Source: CAD feature listing. Evaluate the final solid. Frame: model axes, mm. A direction names the side the tool comes from. Round coordinates to 2 decimals unless told otherwise and drop trailing zeros. Loops run counter-clockwise (first coordinate to the right, second up) from the corner with the lowest first, then second, coordinate; pieces in that order, holes last. Notation, with made-up numbers: (55.5, -31) -> (90.5, -31) arc R38 cw to (90.5, 7) -> close; hole circle Ø6 at (38.25, 81). An arc over 180 degrees is marked (long way). Put each result on its own line as item: value. Start each with the question number.
1. Cut plane A-A (z = 0). Return the cut outline in (x, y), then the cut area to 3 significant figures.
2. Material intervals for L1, parallel to Y at x = 4, z = -4.5; L2, parallel to Z at x = 0, y = 53; L3, parallel to X at y = 32, z = 4.25, sorted ascending.
3. Draft query along Z for faces 1 (the flat face through (20.75, 2, 0)), 2 (the flat face through (10, 2, -10)), 3 (the flat face through (10, 4, 0)). Return one class per face: pulls with the +Z half, pulls with the -Z half, needs draft (parallel to the pull), parting line crosses it, or undercut.
4. Cut plane B-B (x = 0). Return the cut outline in (y, z).
5. Cut plane C-C (z = -7.75). Return the cut outline in (x, y), then the cut area to 3 significant figures.
6. Set-up query: faces 4 (the flat face through (27.25, 2, 0)), 5 (the cylindrical face through (-2.192, 31.608, 4.214)), 6 (the flat face through (16.75, 2, 0)). Return all of +Z, -Z, +X, -X, +Y, -Y with unobstructed straight access to the full face (end or side cutting, diameter ignored); none if empty.
7. Cut plane D-D (y = 8.5). Return the cut outline in (x, z).
8. Contact query for flat-ended pins moving along their axis: pin 1 (3 mm diameter, centred on y = 22, z = -1, fed in from +X); pin 2 (8 mm diameter, centred on x = 0.5, y = 9.5, fed in from -Z); pin 3 (2 mm diameter, centred on y = 47, z = -7.5, fed in from -X); pin 4 (6 mm diameter, centred on y = 43.5, z = -1.5, fed in from -X). Output: stop coordinate, or through.
Autodesk Inventor part; units mm, degrees
ref_plane "YZ Plane" through (0, 0, 0) normal (1, 0, 0) x (0, 1, 0)
ref_plane "XZ Plane" through (0, 0, 0) normal (0, 1, 0) x (-1, 0, 0)
ref_plane "XY Plane" through (0, 0, 0) normal (0, 0, 1) x (1, 0, 0)
sketch "Sketch1" plane through (0, 0, 0) normal (0, 1, 0) x (-1, 0, 0)
  circle A0 centre (0, 0) radius 4.75
  line L0 (7.75, 0) -> (7.75, -10)
  line L1 (7.75, -10) -> (-27.25, -10)
  line L2 (-27.25, -10) -> (-27.25, 10)
  line L3 (-27.25, 10) -> (7.75, 10)
  line L4 (7.75, 10) -> (7.75, 0)
  line L5 (-4.75, 0) -> (-16.75, 0)
  line L6 (-16.75, -10) -> (-16.75, -8.8)
  line L7 (-16.75, 10) -> (-16.75, 8.8)
  line L8 (-16.75, 8.8) -> (-16.75, -8.8)
  line L9 (-16.75, -8.8) -> (-20.75, -8.8)
  line L10 (-20.75, -8.8) -> (-20.75, 8.8)
  line L11 (-20.75, 8.8) -> (-16.75, 8.8)
  line L12 (-20.75, -8.8) -> (-20.75, -10)
  line L13 (-20.75, 8.8) -> (-20.75, 10)
  dimension "d0" = 9.5
  dimension "d2" = 10
  dimension "d3" = 35
  dimension "d4" = 20
  dimension "d5" = 12
  dimension "d6" = 1.2
  dimension "d7" = 1.2
  dimension "d8" = 4
extrude "Extrusion1" add sketch "Sketch1" along normal blind 60 contours A0
extrude "Extrusion2" add sketch "Sketch1" along normal blind 4 contours L8 L7 L3 L4 L0 L1 L6
extrude "Extrusion3" add sketch "Sketch1" along normal blind 4 contours L6 L1 L12 L9
extrude "Extrusion4" add sketch "Sketch1" along normal blind 4 contours L11 L13 L3 L7
extrude "Extrusion5" add sketch "Sketch1" along normal blind 4 contours L10 L12 L1 L2 L3 L13
properties part number "Bluetooth__Base"
Solution:
1. outline: (-7.75, 0) -> (16.75, 0) -> (16.75, 4) -> (4.75, 4) -> (4.75, 60) -> (-4.75, 60) -> (-4.75, 4) -> (-7.75, 4) -> close; (20.75, 0) -> (27.25, 0) -> (27.25, 4) -> (20.75, 4) -> close
1. area: 656 mm^2
2. L1: y = 0 to 4
2. L2: z = -4.75 to 4.75
2. L3: x = -2.12 to 2.12
3. face 1: undercut
3. face 2: pulls with the -Z half
3. face 3: needs draft
4. outline: (0, -10) -> (4, -10) -> (4, -4.75) -> (60, -4.75) -> (60, 4.75) -> (4, 4.75) -> (4, 10) -> (0, 10) -> close
5. outline: (-7.75, 0) -> (16.75, 0) -> (16.75, 4) -> (-7.75, 4) -> close; (20.75, 0) -> (27.25, 0) -> (27.25, 4) -> (20.75, 4) -> close
5. area: 124 mm^2
6. face 4: +Z, -Z, +X, +Y, -Y
6. face 5: +Y
6. face 6: +Y, -Y
7. outline: circle Ø9.5 at (0, 0)
8. pin 1: stops at x = 4.75
8. pin 2: stops at z = -4.75
8. pin 3: passes through
8. pin 4: stops at x = -4.75
